Study the drawing (mm; zero at the part's minimum x, y, z) and answer. Coordinates: 2 decimals unless noted, no trailing zeros. Order: outer loops, then holes, each group sorted by start corner. A loop starts at its lowest first (then second) coordinate and runs counter-clockwise, first axis right, second up.
1. The part is cut by section B-B, the plane y = 207.5. Give the vertices of the cut face in (x, z) (1 decimal).
2. The part is cut by section C-C, the plane x = 32.5. Give the vertices of the cut face in (y, z) (1 decimal).
3. The part is cut by section A-A, the plane x = 130. Give the vertices of the cut face in (y, z).
4. The part is cut by section D-D, the plane z = 6.75. Count the separate pieces of the cut face and the enclosed holes in it, then the cut area to 3 significant figures.
5. Flat-ended cylindrical pins translate along their axes: pin 1 Ø1 at (y, z) = (188, 11.5) entering from +X; pin 2 Ø1 at (y, z) = (229.5, 11.5) entering from -X; pin 3 Ø1.5 at (x, z) = (56, 9) entering from +Y. Find the tip coordinate at first contact, or state that the pin passes through.
6. Find the intervals of material crossed by probe 1 along X at (y, z) = (29, 1.25); probe 2 along Y at (x, z) = (130, 12.75); probe 3 along Y at (x, z) = (100, 4.25) (1 decimal), in increasing order.
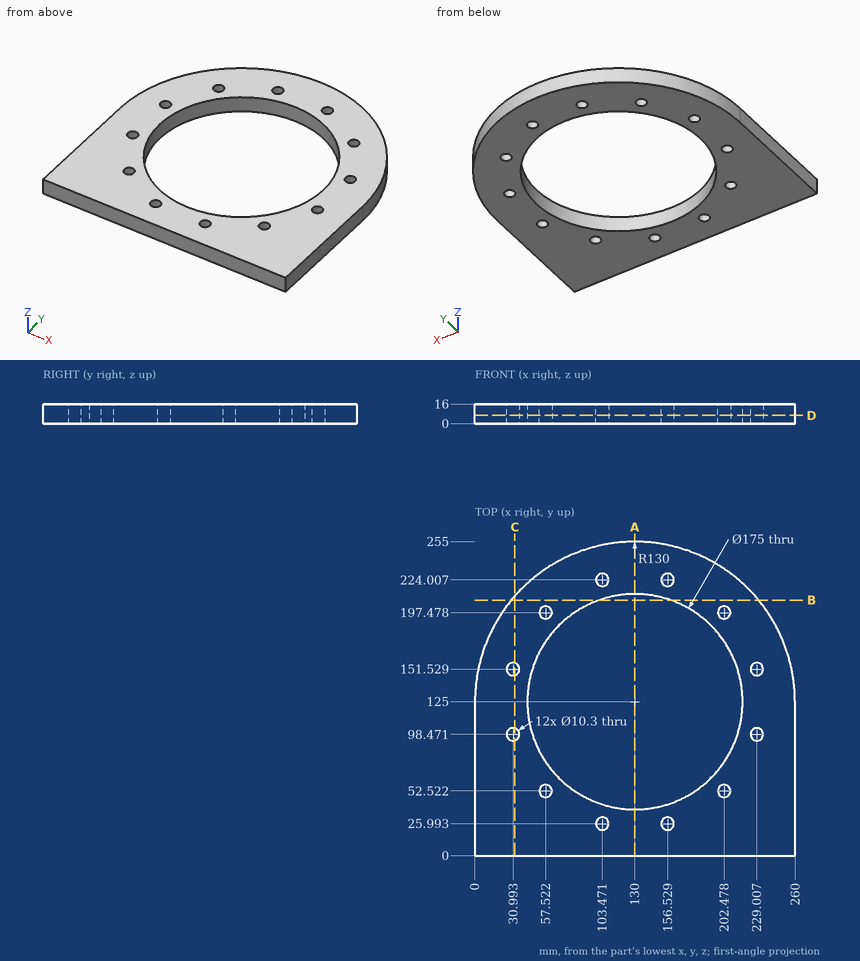
Geometry says:
1. outline: (29.5, 0) - (100.8, 0) - (100.8, 16) - (29.5, 16) - close; (159.2, 0) - (230.5, 0) - (230.5, 16) - (159.2, 16) - close
2. outline: (0, 0) - (93.5, 0) - (93.5, 16) - (0, 16) - close; (103.4, 0) - (146.6, 0) - (146.6, 16) - (103.4, 16) - close; (156.5, 0) - (211, 0) - (211, 16) - (156.5, 16) - close
3. outline: (0, 0) - (37.5, 0) - (37.5, 16) - (0, 16) - close; (212.5, 0) - (255, 0) - (255, 16) - (212.5, 16) - close
4. separate pieces: 1
4. enclosed holes: 13
4. area: 34,000 mm2
5. pin 1: stops at x = 243.99
5. pin 2: stops at x = 52
5. pin 3: stops at y = 232.4
6. probe 1: x = 0 to 99.29, 107.65 to 152.35, 160.71 to 260
6. probe 2: y = 0 to 37.5, 212.5 to 255
6. probe 3: y = 0 to 22.2, 29.8 to 42.8, 207.2 to 220.2, 227.8 to 251.5
